from build123d import *

# Parameters (mm, degrees)
SKETCH1_R           = 2.8575
BOSS_EXTRUDE1_DEPTH = 3.5052
CUT_EXTRUDE1_DEPTH  = 1.9558
SKETCH3_R           = 1.7145
BOSS_EXTRUDE2_DEPTH = 4.7625


with BuildPart() as part:
    # Sketch1 → Boss-Extrude1 (new body)
    with BuildSketch(Plane(origin=(0, 0, 0), x_dir=(1, 0, 0), z_dir=(0, 1, 0))):
        Circle(SKETCH1_R)
    extrude(amount=BOSS_EXTRUDE1_DEPTH)

    # Sketch2 → Cut-Extrude1 (cut)
    with BuildSketch(Plane.XZ):
        Polygon((1.603951217, 0), (0.801975608, 1.3890625), (-0.801975608, 1.3890625), (-1.603951217, 0), (-0.801975608, -1.3890625), (0.801975608, -1.3890625), align=None)
    extrude(amount=-CUT_EXTRUDE1_DEPTH, mode=Mode.SUBTRACT)

    # Sketch3 → Boss-Extrude2 (add)
    with BuildSketch(Plane(origin=(0, 3.5052, 0), x_dir=(1, 0, 0), z_dir=(0, 1, 0))):
        Circle(SKETCH3_R)
    extrude(amount=BOSS_EXTRUDE2_DEPTH)


solid = part.part
Here's how the part is built. I have some questions about the finished solid (model axes, mm). A direction names the side the tool comes from. Give positions to 0.01 mm unless a question says otherwise; leave off trailing zeros. Write each loop counter-clockwise with the first axis right and the second up, starting at its lowest first coordinate (ties: lowest second). Pieces come first, ordered by that corner, then holes. Notation, with made-up numbers: (13.5, 22.25) -> (18.5, 22.25) arc R13 ccw to (18.5, 40.25) -> close; hole circle Ø1 at (29.25, 41). An arc over 180 degrees is marked (long way). Use one line per item in the form item = value. Start each with the question number.
1. Imagine slicing it at D-D on z = -1.95. List the corners of the cut face in (x, y) for me, plus the area to 3 significant figures.
2. Thinking about a two-plate mould opening in Z: for faces 4 (the face through (2.726, 1.728, -0.858)), 5 (the face through (0, 3.505, 2)), 6 (the face through (-1.2, 1, -0.7)), which applies, +Z half, -Z half, draft (parallel to the pull), parting line (faces both ways), or undercut?
3. Will these pins go through, and if not, where does the flat tip stop? pin 1 Ø3 at (x, y) = (-1.5, 5.5) entering from +Z; pin 2 Ø2 at (x, z) = (-0.5, -0.5) entering from -Y.
4. Imagine slicing it at B-B on y = 5. List the corners of the cut face in (x, z) for me, plus the area to 3 significant figures.
5. On a 3-axis mill with a long thin cutter (end or side, diameter ignored), from which of +Z, -Z, +X, -X, +Y, -Y can I reach the whole of each face in a straight line? I mean faces 1 (the face through (1.2, 1, 0.7)), 2 (the face through (0, 8.268, 0)), 3 (the face through (-0.372, 5.853, 1.674)). Say none if no direction works.
6. If I drill on L1, parallel to Y at x = 1.9, z = 0.75; L2, parallel to Y at x = 0.35, z = 0.55; L3, parallel to Z at x = -0.8, y = 7.5, over which ranges is the centre line in solid material (lowest first)?
7. Imagine slicing it at A-A on x = 0. List the corners of the cut face in (y, z) for me.
8. Imagine slicing it at C-C on x = 1.45. List the corners of the cut face in (y, z) for me.
Entries:
q1.outline = (-2.09, 0) -> (2.09, 0) -> (2.09, 3.51) -> (-2.09, 3.51) -> close
q1.area = 14.6 mm²
q2.face_4 = parting line
q2.face_5 = draft
q2.face_6 = undercut
q3.pin_1 = 1.71
q3.pin_2 = 0
q4.outline = circle Ø3.43 at (0, 0)
q4.area = 9.23 mm²
q5.face_1 = -Y
q5.face_2 = +Z, -Z, +X, -X, +Y
q5.face_3 = +Y
q6.L1 = 0 to 3.51
q6.L2 = 1.96 to 8.27
q6.L3 = -1.52 to 1.52
q7.outline = (0, -2.86) -> (3.51, -2.86) -> (3.51, -1.71) -> (8.27, -1.71) -> (8.27, 1.71) -> (3.51, 1.71) -> (3.51, 2.86) -> (0, 2.86) -> (0, 1.39) -> (1.96, 1.39) -> (1.96, -1.39) -> (0, -1.39) -> close
q8.outline = (0, -2.46) -> (3.51, -2.46) -> (3.51, -0.91) -> (8.27, -0.91) -> (8.27, 0.91) -> (3.51, 0.91) -> (3.51, 2.46) -> (0, 2.46) -> (0, 0.27) -> (1.96, 0.27) -> (1.96, -0.27) -> (0, -0.27) -> close
